Here's how the part is built. I have some questions about the finished solid (model axes, mm). Round coordinates to 2 decimals unless told otherwise and drop trailing zeros. Loops run counter-clockwise (first coordinate to the right, second up) from the corner with the lowest first, then second, coordinate; pieces in that order, holes last. Notation, with made-up numbers: (15, -32.75) -> (29, -32.75) arc R31 ccw to (29, -6.75) -> close; hole circle Ø3 at (32.5, -23.75). An arc over 180 degrees is marked (long way). One line per item, written item: value. Start each with the question number.
```python
from build123d import *

# Parameters (mm, degrees)
SKETCH1_W           = 220.98
SKETCH1_H           = 256.54
BOSS_EXTRUDE1_DEPTH = 5.08
FILLET1_R           = 5.08
FILLET2_R           = 5.08
SKETCH2_R           = 1.27
BOSS_EXTRUDE2_DEPTH = 6.35


# Some blends are built 0.0001 mm under size
with BuildPart() as part:
    # Sketch1 → Boss-Extrude1 (new body)
    with BuildSketch(Plane.XY):
        with Locations((110.49, 128.27)):
            Rectangle(SKETCH1_W, SKETCH1_H)
    extrude(amount=BOSS_EXTRUDE1_DEPTH)

    # Fillet1
    fillet1_edges = [part.edges().sort_by_distance(p)[0] for p in [
        (110.49, 0, 5.08),
        (220.98, 128.27, 5.08),
        (0, 128.27, 5.08),
        (110.49, 256.54, 5.08),
    ]]
    fillet(fillet1_edges, radius=FILLET1_R - 0.0001)  # a hair under: the kernel refuses the full size

    # Fillet2
    # the kernel refuses this fillet: 5.08 mm, written as the material it takes off along each edge
    with BuildSketch(Plane(origin=(5.08, 251.46, 5.08), x_dir=(0, 1, 0), z_dir=(1, 0, 0))) as fillet2_piece_1:
        with BuildLine():
            CenterArc((0.0001, -5.0799), 5.0799, 0, 90)
            Line((5.08, -5.0799), (5.08, 0))
            Line((5.08, 0), (0.0001, 0))
        make_face()
    revolve(axis=Axis((5.08, 251.46, 5.08), (0, 0, 1)), revolution_arc=90, mode=Mode.SUBTRACT)
    with BuildSketch(Plane(origin=(215.9, 251.46, 5.08), x_dir=(1, 0, 0), z_dir=(0, -1, 0))) as fillet2_piece_2:
        with BuildLine():
            CenterArc((0.0001, -5.0799), 5.0799, 0, 90)
            Line((5.08, -5.0799), (5.08, 0))
            Line((5.08, 0), (0.0001, 0))
        make_face()
    revolve(axis=Axis((215.9, 251.46, 5.08), (0, 0, 1)), revolution_arc=90, mode=Mode.SUBTRACT)
    with BuildSketch(Plane(origin=(5.08, 5.08, 5.08), x_dir=(-1, 0, 0), z_dir=(0, 1, 0))) as fillet2_piece_3:
        with BuildLine():
            CenterArc((0.0001, -5.0799), 5.0799, 0, 90)
            Line((5.08, -5.0799), (5.08, 0))
            Line((5.08, 0), (0.0001, 0))
        make_face()
    revolve(axis=Axis((5.08, 5.08, 5.08), (0, 0, 1)), revolution_arc=90, mode=Mode.SUBTRACT)
    with BuildSketch(Plane(origin=(215.9, 5.08, 5.08), x_dir=(0, -1, 0), z_dir=(-1, 0, 0))) as fillet2_piece_4:
        with BuildLine():
            CenterArc((0.0001, -5.0799), 5.0799, 0, 90)
            Line((5.08, -5.0799), (5.08, 0))
            Line((5.08, 0), (0.0001, 0))
        make_face()
    revolve(axis=Axis((215.9, 5.08, 5.08), (0, 0, 1)), revolution_arc=90, mode=Mode.SUBTRACT)
    with BuildSketch(Plane(origin=(220.98, 0, -12.7), x_dir=(-1, 0, 0), z_dir=(0, 0, 1)), Plane(origin=(220.98, 256.54, -12.7), x_dir=(0, -1, 0), z_dir=(0, 0, 1))) as fillet2_piece_5:
        with BuildLine():
            CenterArc((FILLET2_R, -FILLET2_R), FILLET2_R, 90, 90)
            Line((0, -FILLET2_R), (0, 0))
            Line((0, 0), (FILLET2_R, 0))
        make_face()
    extrude(amount=17.78, mode=Mode.SUBTRACT)
    with BuildSketch(Plane(origin=(0, 0, -12.7), x_dir=(1, 0, 0), z_dir=(0, 0, 1)), Plane(origin=(0, 256.54, -12.7), x_dir=(0, -1, 0), z_dir=(0, 0, 1))) as fillet2_piece_6:
        with BuildLine():
            CenterArc((FILLET2_R, FILLET2_R), FILLET2_R, 180, 90)
            Line((0, FILLET2_R), (0, 0))
            Line((0, 0), (FILLET2_R, 0))
        make_face()
    extrude(amount=17.78, mode=Mode.SUBTRACT)

    # Sketch2 → Boss-Extrude2 (add)
    with BuildSketch(Plane(origin=(0, 0, 0), x_dir=(-1, 0, 0), z_dir=(0, 0, -1))):
        with Locations((-213.0425, 248.6025)):
            Circle(SKETCH2_R)
        with Locations((-7.9375, 248.6025)):
            Circle(SKETCH2_R)
        with Locations((-213.0425, 7.9375)):
            Circle(SKETCH2_R)
        with Locations((-7.9375, 7.9375)):
            Circle(SKETCH2_R)
    extrude(amount=BOSS_EXTRUDE2_DEPTH)


solid = part.part
```
Q1. If I drill on line 1 along Z through (x, y) = (63, 37.5); line 2 along Y through (x, z) = (9, -3.5); line 3 along X through (y, z) = (135.5, 0.75), over which ranges is the centre line in solid material (lowest first)?
Q2. I want a section at C-C on z = -3.75. Please give me the cut outline in (x, y), plus the area to 3 significant figures.
Q3. Will these pins go through, and if not, where does the flat tip stop? P1, Ø4, axis at x = 162.5, y = 145.5, coming from the -Z side; P2, Ø1.5, axis at y = 135, z = 2, coming from the +X side; P3, Ø6, axis at y = 48.5, z = 0.5, coming from the -X side.
Answers below:
1. line 1: z = 0 to 5.08
1. line 2: y = 7.24 to 8.63, 247.91 to 249.3
1. line 3: x = 0.06 to 220.92
2. outline: circle Ø2.54 at (7.94, 7.94); circle Ø2.54 at (7.94, 248.6); circle Ø2.54 at (213.04, 7.94); circle Ø2.54 at (213.04, 248.6)
2. area: 20.3 mm^2
3. P1: stops at z = 0
3. P2: stops at x = 220.82
3. P3: stops at x = 0
